Geometry check sheet. Reference: the model listing, model coordinates, mm. Face numbers are marked on the shaded views. A direction names the side the tool comes from. Round coordinates to 2 decimals unless told otherwise and drop trailing zeros. Order: outer loops, then holes, each group sorted by start corner. A loop starts at its lowest first (then second) coordinate and runs counter-clockwise, first axis right, second up.
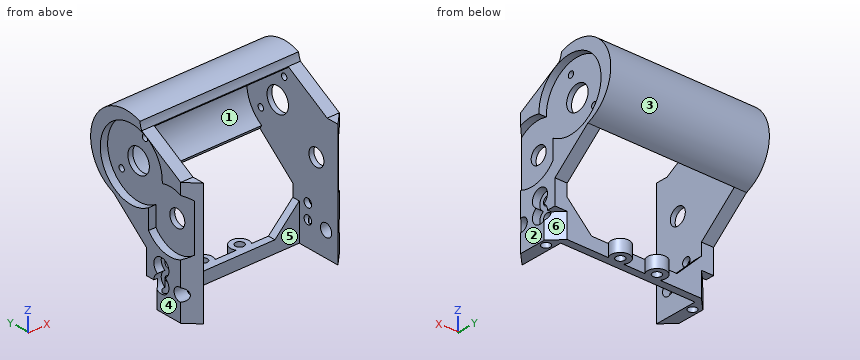
```python
from build123d import *

# Parameters (mm, degrees)
SKETCH1_R           = 5
SKETCH1_R_2         = 1.25
SKETCH1_R_3         = 3.5
SKETCH1_R_4         = 1.75
SKETCH1_R_5         = 2.6
BOSS_EXTRUDE1_DEPTH = 5
CUT_EXTRUDE12_DEPTH = 3
CUT_EXTRUDE15_REACH = 72.749
BOSS_EXTRUDE2_START = -65
SKETCH7_W           = 5
SKETCH7_H           = 3
BOSS_EXTRUDE2_DEPTH = 65
SKETCH8_R           = 1.75
CUT_EXTRUDE16_DEPTH = 10
SKETCH10_R          = 3.75
SKETCH10_R_2        = 1.75
BOSS_EXTRUDE3_DEPTH = 5
CHAMFER1_SIZE       = 10


with BuildPart() as part:
    # Sketch1 → Boss-Extrude1 (new body)
    with BuildSketch(Plane(origin=(0, 0, 0), x_dir=(0, 0, -1), z_dir=(1, 0, 0))):
        with BuildLine():
            Line((-3.451085907, -28.022543867), (46.548914093, -28.022543867))
            Line((46.548914093, -28.022543867), (46.548914093, -7.022543867))
            Line((46.548914093, -7.022543867), (26.548914093, -7.022543867))
            Line((26.548914093, -7.022543867), (13.706594967, 8.30960665))
            ThreePointArc((13.706594967, 8.30960665), (-7.876735811, 17.766067564), (-16.904643834, -4))
            ThreePointArc((-16.904643834, -4), (-15.383939757, -4.319460395), (-13.931085907, -4.870651404))
            Line((-13.931085907, -4.870651404), (-3.451085907, -23.022543867))
            Line((-3.451085907, -23.022543867), (-3.451085907, -28.022543867))
        make_face()
        Circle(SKETCH1_R, mode=Mode.SUBTRACT)
        with Locations((6.061215112, 7.906432278)):
            Circle(SKETCH1_R_2, mode=Mode.SUBTRACT)
        with Locations((-9.50267373, -2.991520012)):
            Circle(SKETCH1_R_2, mode=Mode.SUBTRACT)
        with Locations((12.6186816, -18.021344974)):
            Circle(SKETCH1_R_3, mode=Mode.SUBTRACT)
        with Locations((36.548914093, -14.022543867)):
            Circle(SKETCH1_R_4, mode=Mode.SUBTRACT)
        with Locations((30.548914093, -14.022543867)):
            Circle(SKETCH1_R_4, mode=Mode.SUBTRACT)
        with Locations((36.548914093, -22.522543867)):
            Circle(SKETCH1_R_5, mode=Mode.SUBTRACT)
    boss_extrude1 = extrude(amount=BOSS_EXTRUDE1_DEPTH)

    # Sketch2 → Cut-Extrude12 (cut)
    with BuildSketch(Plane(origin=(5, 0, 0), x_dir=(0, 0, -1), z_dir=(1, 0, 0))):
        with BuildLine():
            Line((9.1186816, -30.021344974), (16.1186816, -30.021344974))
            ThreePointArc((16.1186816, -30.021344974), (24.917055476, -20.257412952), (20.1186816, -8.021344974))
            Line((20.1186816, -8.021344974), (12.019173216, -8.021344974))
            ThreePointArc((12.019173216, -8.021344974), (-7.097524936, 12.586804193), (0.644011182, -14.435641641))
            ThreePointArc((0.644011182, -14.435641641), (1.637110982, -23.992534703), (9.1186816, -30.021344974))
        make_face()
        with BuildLine():
            ThreePointArc((33.548914093, -15.825319505), (40.048914093, -14.022543867), (33.548914093, -12.219768229))
            ThreePointArc((33.548914093, -12.219768229), (27.048914093, -14.022543867), (33.548914093, -15.825319505))
        make_face()
    cut_extrude12 = extrude(amount=-CUT_EXTRUDE12_DEPTH, mode=Mode.SUBTRACT)

    # Sketch6 → Cut-Extrude15 (cut, up to next)
    with BuildSketch(Plane(origin=(0, 0, -46.548914093), x_dir=(-1, 0, 0), z_dir=(0, 0, -1)), mode=Mode.PRIVATE) as cut_extrude15_sk1:
        Polygon((0, -28.022543867), (-5, -23.022543867), (-6.777242855, -29.799786723), align=None)
    cut_extrude15_tool1 = extrude(cut_extrude15_sk1.sketch, amount=-CUT_EXTRUDE15_REACH, mode=Mode.PRIVATE) & part.part
    cut_extrude15 = cut_extrude15_tool1.solids().sort_by_distance((3.925748, -26.948291, -46.548914))[0]
    add(cut_extrude15, mode=Mode.SUBTRACT)

    # Sketch7 → Boss-Extrude2 (add)
    with BuildSketch(Plane(origin=(5, 0, 0), x_dir=(0, 0, -1), z_dir=(1, 0, 0)).offset(BOSS_EXTRUDE2_START)):
        with BuildLine():
            Line((-13.931085907, -4.870651404), (-13.604383665, -4.870651404))
            ThreePointArc((-13.604383665, -4.870651404), (-6.212314592, 13.046441944), (12.35657784, 7.491160397))
            Line((12.35657784, 7.491160397), (13.706594967, 8.30960665))
            ThreePointArc((13.706594967, 8.30960665), (-7.876735811, 17.766067564), (-16.904643834, -4))
            ThreePointArc((-16.904643834, -4), (-15.383939757, -4.319460395), (-13.931085907, -4.870651404))
        make_face()
        with Locations((44.048914093, -8.522543867)):
            Rectangle(SKETCH7_W, SKETCH7_H)
    extrude(amount=BOSS_EXTRUDE2_DEPTH)

    # Mirror4: Boss-Extrude1, Cut-Extrude12, Cut-Extrude15 across plane
    add(boss_extrude1.mirror(Plane(origin=(-27.5, 0, 0), x_dir=(0, 0, 1), z_dir=(1, 0, 0))))
    add(cut_extrude12.mirror(Plane(origin=(-27.5, 0, 0), x_dir=(0, 0, 1), z_dir=(1, 0, 0))), mode=Mode.SUBTRACT)
    add(cut_extrude15.mirror(Plane(origin=(-27.5, 0, 0), x_dir=(0, 0, 1), z_dir=(1, 0, 0))), mode=Mode.SUBTRACT)

    # Sketch8 → Cut-Extrude16 (cut)
    with BuildSketch(Plane(origin=(0, 0, -46.548914093), x_dir=(-1, 0, 0), z_dir=(0, 0, -1))):
        with Locations(Location((-2.5, -14.022543867, 0), (0, 0, 90))):
            Circle(SKETCH8_R)
        with Locations(Location((57.5, -14.022543867, 0), (0, 0, 90))):
            Circle(SKETCH8_R)
        Polygon((55, -7.022543867), (60, -12.022543867), (62.67758006, -4.344963807), align=None)
        Polygon((0, -7.022543867), (-5, -12.022543867), (-6.777064695, -5.245479172), align=None)
    extrude(amount=-CUT_EXTRUDE16_DEPTH, mode=Mode.SUBTRACT)

    # Sketch10 → Boss-Extrude3 (add)
    # profile 1 of 2: a face of its own
    with BuildSketch(Plane(origin=(0, 0, -46.548914093), x_dir=(-1, 0, 0), z_dir=(0, 0, -1))):
        with Locations((35, -5.022543867)):
            Circle(SKETCH10_R)
        with Locations(Location((35, -5.022543867, 0), (0, 0, 90))):
            Circle(SKETCH10_R_2, mode=Mode.SUBTRACT)
    # profile 2 of 2: a face of its own
    with BuildSketch(Plane(origin=(0, 0, -46.548914093), x_dir=(-1, 0, 0), z_dir=(0, 0, -1))):
        with Locations((20, -5.022543867)):
            Circle(SKETCH10_R)
        with Locations(Location((20, -5.022543867, 0), (0, 0, 90))):
            Circle(SKETCH10_R_2, mode=Mode.SUBTRACT)
    extrude(amount=-BOSS_EXTRUDE3_DEPTH)

    # Chamfer1
    # the kernel refuses this chamfer: 10 mm, written as the material it adds along each edge
    with BuildSketch(Plane(origin=(0, -10.022543867, -41.548914093), x_dir=(-0.9996219169112968, 0, -0.027495876610586317), z_dir=(0, 1, 0)), Plane(origin=(-55, -7.022543867, -41.548914093), x_dir=(0.9996219169112968, 0, -0.027495876610586317), z_dir=(0, -1, 0))) as chamfer1_piece_1:
        Polygon((CHAMFER1_SIZE * 0.999621916911, CHAMFER1_SIZE * 0.0274958766106), (-CHAMFER1_SIZE * 0.0274958766106, CHAMFER1_SIZE * 0.999621916911), (0, 0), align=None)
    extrude(amount=3)


solid = part.part
```
(1) Set-up check for the marked faces 4, 5 and 6: record each of +Z, -Z, +X, -X, +Y, -Y from which the full face is reachable in a straight line by a thin tool's end or side.
Returned:
face 4: +Z, -Z, -X, +Y, -Y
face 5: +Z, -Z, -Y
face 6: -Z, +X, +Y
(2) Sectioned sample at C-C, the plane y = 12. Record the cut outline in (x, z).
Returned:
outline: (-60, -11.74) - (5, -11.74) - (5, -8.05) - (2, -8.05) - (2, 8.05) - (5, 8.05) - (5, 15.18) - (-60, 15.18) - (-60, 8.05) - (-57, 8.05) - (-57, -8.05) - (-60, -8.05) - close; hole (-55, -8.05) - (0, -8.05) - (0, 8.05) - (-55, 8.05) - close
(3) Sectioned sample at A-A, the plane x = -12. Record the cut outline in (y, z), and give its area (3 significant figures).
Returned:
outline: (-10.02, -46.55) - (-7.02, -46.55) - (-7.02, -41.55) - (-10.02, -41.55) - close; (-4.87, 13.6) arc R14.45 cw to (7.49, -12.36) - (8.31, -13.71) arc R16.5 ccw (long way) to (-4, 16.9) arc R10 cw to (-4.87, 13.93) - close
area: 203 mm2
(4) Draft check along Z on the marked faces 1, 2 and 3. Enter one of: released by +Z, released by -Z, zero draft, split by the parting line, or undercut.
Returned:
face 1: undercut
face 2: zero draft
face 3: split by the parting line
(5) Material ranges on line 1 (X direction, y = 3.5, z = 5); line 2 (X direction, y = -18, z = -39.5); line 3 (Z direction, x = 0.9, y = 0), recorded low to high.
Returned:
line 1: x = -57 to -55, 0 to 2
line 2: x = -60 to -55, 0 to 5
line 3: z = -20.67 to -5, 5 to 18.04
(6) Sectioned sample at B-B, the plane y = 0. Record the cut outline in (x, z), and give its area (3 significant figures).
Returned:
outline: (-60, -20.67) - (-55, -20.67) - (-55, -5) - (-57, -5) - (-57, -14.45) - (-60, -14.45) - close; (-60, 14.45) - (-57, 14.45) - (-57, 5) - (-55, 5) - (-55, 14.45) - (0, 14.45) - (0, 5) - (2, 5) - (2, 14.45) - (5, 14.45) - (5, 18.04) - (-60, 18.04) - close; (0, -20.67) - (5, -20.67) - (5, -14.45) - (2, -14.45) - (2, -5) - (0, -5) - close
area: 371 mm2
(7) Depth check by flat-ended pin: P1, Ø3, axis at y = -14.02, z = -30.55, coming from the -X side; P2, Ø5.5, axis at y = -14.02, z = -36.55, coming from the +X side; P3, Ø2, axis at x = -19, y = -2.5, coming from the +Z side; P4, Ø3, axis at x = -57.5, y = -14.02, coming from the -Z side. Enter the tip coordinate at first touch or a pass-through.
Returned:
P1: passes through
P2: stops at x = 2
P3: stops at z = 17.74
P4: stops at z = -35.52
